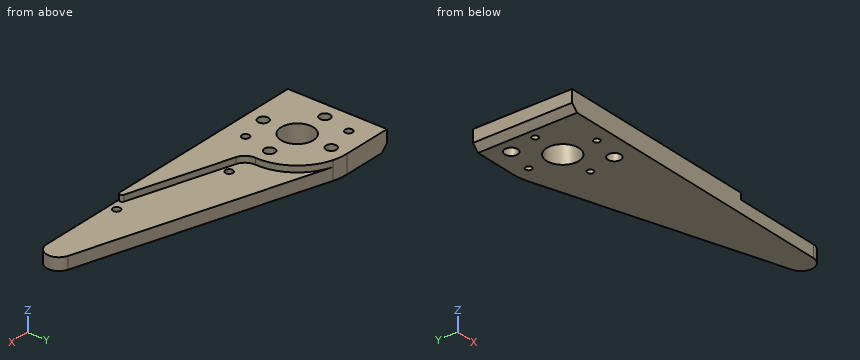
```python
from build123d import *

# Parameters (mm, degrees)
ESTRUSIONE1_DEPTH        = 15
SMUSSO1_SIZE             = 5
SCHIZZO2_R               = 13
TAGLIO_ESTRUSIONE1_DEPTH = 59.523499554
SCHIZZO4_R               = 3
TAGLIO_ESTRUSIONE3_DEPTH = 20
SCHIZZO5_R               = 5.25
TAGLIO_ESTRUSIONE4_DEPTH = 8.5
SCHIZZO6_R               = 2.5
TAGLIO_ESTRUSIONE5_DEPTH = 20
SCHIZZO7_R               = 4.25
TAGLIO_ESTRUSIONE6_DEPTH = 6
ESTRUSIONE2_START        = -15
ESTRUSIONE2_DEPTH        = 15
TAGLIO_ESTRUSIONE7_START = -5
TAGLIO_ESTRUSIONE7_DEPTH = 5
SCHIZZO10_R              = 3
TAGLIO_ESTRUSIONE8_DEPTH = 10
RACCORDO1_R              = 2


with BuildPart() as part:
    # Schizzo1 → Estrusione1 (new body)
    with BuildSketch(Plane.XY):
        with BuildLine():
            Line((-40, 40), (0, 40))
            ThreePointArc((0, 40), (40, 0), (0, -40))
            Line((0, -40), (-40, -40))
            Line((-40, -40), (-40, 40))
        make_face()
    extrude(amount=ESTRUSIONE1_DEPTH)

    # Smusso1
    smusso1_edges = [part.edges().sort_by_distance(p)[0] for p in [
        (-40, 0, 0),
    ]]
    chamfer(smusso1_edges, length=SMUSSO1_SIZE)

    # Schizzo2 → Taglio-Estrusione1 (cut, through all)
    with BuildSketch(Plane(origin=(0, 0, 0), x_dir=(-1, 0, 0), z_dir=(0, 0, -1))):
        Circle(SCHIZZO2_R)
    extrude(amount=-TAGLIO_ESTRUSIONE1_DEPTH, mode=Mode.SUBTRACT)

    # Schizzo4 → Taglio-Estrusione3 (cut)
    with BuildSketch(Plane.XY.offset(15)):
        with Locations((-22.980970389, 22.980970389)):
            Circle(SCHIZZO4_R)
        with Locations((22.980970389, -22.980970389)):
            Circle(SCHIZZO4_R)
    extrude(amount=-TAGLIO_ESTRUSIONE3_DEPTH, mode=Mode.SUBTRACT)

    # Schizzo5 → Taglio-Estrusione4 (cut)
    with BuildSketch(Plane.XY):
        with Locations((-22.980970389, 22.980970389)):
            Circle(SCHIZZO5_R)
        with Locations(Location((22.980970389, -22.980970389, 0), (0, 0, 180))):
            Circle(SCHIZZO5_R)
    extrude(amount=TAGLIO_ESTRUSIONE4_DEPTH, mode=Mode.SUBTRACT)

    # Schizzo6 → Taglio-Estrusione5 (cut)
    with BuildSketch(Plane(origin=(0, 0, 0), x_dir=(-1, 0, 0), z_dir=(0, 0, -1))):
        with Locations((27.5, 0)):
            Circle(SCHIZZO6_R)
        with Locations((0, -27.5)):
            Circle(SCHIZZO6_R)
        with Locations((-27.5, 0)):
            Circle(SCHIZZO6_R)
        with Locations((0, 27.5)):
            Circle(SCHIZZO6_R)
    extrude(amount=-TAGLIO_ESTRUSIONE5_DEPTH, mode=Mode.SUBTRACT)

    # Schizzo7 → Taglio-Estrusione6 (cut)
    with BuildSketch(Plane.XY.offset(15)):
        with Locations((0, 27.5)):
            Circle(SCHIZZO7_R)
        with Locations((-27.5, 0)):
            Circle(SCHIZZO7_R)
        with Locations((27.5, 0)):
            Circle(SCHIZZO7_R)
        with Locations((0, -27.5)):
            Circle(SCHIZZO7_R)
    extrude(amount=-TAGLIO_ESTRUSIONE6_DEPTH, mode=Mode.SUBTRACT)

    # Schizzo8 → Estrusione2 (add)
    with BuildSketch(Plane.XY.offset(15).offset(ESTRUSIONE2_START)):
        with BuildLine():
            Line((11.73594132, 38.239608802), (202.93398533, -20.4400978))
            ThreePointArc((202.93398533, -20.4400978), (209.889363529, -31.483404529), (200, -40))
            Line((200, -40), (0, -40))
            ThreePointArc((0, -40), (39.557454115, -5.933618117), (11.73594132, 38.239608802))
        make_face()
    extrude(amount=ESTRUSIONE2_DEPTH)

    # Schizzo9 → Taglio-Estrusione7 (cut)
    with BuildSketch(Plane.XY.offset(15).offset(TAGLIO_ESTRUSIONE7_START)):
        with BuildLine():
            Line((140.558333333, -40), (200, -40))
            ThreePointArc((200, -40), (209.889363529, -31.483404529), (202.93398533, -20.4400978))
            Line((202.93398533, -20.4400978), (11.73594132, 38.239608802))
            ThreePointArc((11.73594132, 38.239608802), (32.5753606, 23.213054125), (39.975840489, -1.390027772))
            ThreePointArc((39.975840489, -1.390027772), (41.825960461, -7.540798246), (47.035815281, -11.297436915))
            Line((47.035815281, -11.297436915), (140.558333333, -40))
        make_face()
    extrude(amount=TAGLIO_ESTRUSIONE7_DEPTH, mode=Mode.SUBTRACT)

    # Schizzo10 → Taglio-Estrusione8 (cut)
    with BuildSketch(Plane.XY.offset(15)):
        with Locations((57, -8.648405099)):
            Circle(SCHIZZO10_R)
        with Locations((138.285904257, -33.5)):
            Circle(SCHIZZO10_R)
    extrude(amount=-TAGLIO_ESTRUSIONE8_DEPTH, mode=Mode.SUBTRACT)

    # Raccordo1
    raccordo1_edges = [part.edges().sort_by_distance(p)[0] for p in [
        (140.558333333, -40, 12.5),
    ]]
    fillet(raccordo1_edges, radius=RACCORDO1_R)


solid = part.part
```
Geometry check sheet. Reference: the model listing, model coordinates, mm. Give positions to 0.01 mm unless a question says otherwise; leave off trailing zeros. Write each loop counter-clockwise with the first axis right and the second up, starting at its lowest first coordinate (ties: lowest second). Pieces come first, ordered by that corner, then holes. Notation, with made-up numbers: (26, 76) -> (55, 76) arc R16 ccw to (55, 90) -> close; hole circle Ø8 at (48, 88). An arc over 180 degrees is marked (long way). Use one line per item in the form item = value.
Item 1: Depth check by flat-ended pin: pin 1 Ø6.5 at (x, y) = (56, -8) entering from +Z; pin 2 Ø1.5 at (y, z) = (0, 13) entering from +X; pin 3 Ø5 at (x, y) = (-24.5, 22.5) entering from -Z. Enter the tip coordinate at first touch or a pass-through.
Results list:
pin_1 = 10
pin_2 = 40
pin_3 = 8.5
Item 2: Sectioned sample at B-B on z = 12.5. Enter the section's corners in (x, y) (3 decimals).
Results list:
outline = (-40, -40) -> (127.225, -40) arc R2 ccw to (127.812, -36.088) -> (47.036, -11.297) arc R10 cw to (39.976, -1.39) arc R40 ccw to (0, 40) -> (-40, 40) -> close; hole circle Ø8.5 at (-27.5, 0); hole circle Ø6 at (-22.981, 22.981); hole circle Ø26 at (0, 0); hole circle Ø8.5 at (0, -27.5); hole circle Ø8.5 at (0, 27.5); hole circle Ø6 at (22.981, -22.981); hole circle Ø8.5 at (27.5, 0)
Item 3: Sectioned sample at A-A on y = 10. Enter the section's corners in (x, z).
Results list:
outline = (-40, 5) -> (-35, 0) -> (-8.31, 0) -> (-8.31, 15) -> (-40, 15) -> close; (8.31, 0) -> (103.75, 0) -> (103.75, 10) -> (38.73, 10) -> (38.73, 15) -> (8.31, 15) -> close
Item 4: Sectioned sample at D-D on x = 57. Enter the section's corners in (y, z), plus the area to 3 significant figures.
Results list:
outline = (-40, 0) -> (24.35, 0) -> (24.35, 10) -> (-5.65, 10) -> (-5.65, 5) -> (-11.65, 5) -> (-11.65, 10) -> (-14.36, 10) -> (-14.36, 15) -> (-40, 15) -> close
area = 742 mm2
Item 5: Sectioned sample at C-C on x = 110. Enter the section's corners in (y, z).
Results list:
outline = (-40, 0) -> (8.08, 0) -> (8.08, 10) -> (-30.62, 10) -> (-30.62, 15) -> (-40, 15) -> close
Item 6: Scan lines: line 1 (Y direction, x = 0, z = 3.25); line 2 (Y direction, x = 0, z = 10.8); line 3 (Y direction, x = 29.5, z = 6). Record each from-to range of solid material in increasing order.
Results list:
line_1 = -40 to -30, -25 to -13, 13 to 25, 30 to 40
line_2 = -40 to -31.75, -23.25 to -13, 13 to 23.25, 31.75 to 40
line_3 = -40 to -1.5, 1.5 to 32.79
